from build123d import *

# Parameters (mm, degrees)
SKETCH_W     = 42
SKETCH_H     = 42
PAD_DEPTH    = 47
SKETCH001_R  = 1.5
POCKET_DEPTH = 4.5
SKETCH002_R  = 11
PAD001_DEPTH = 2
SKETCH003_R  = 2.5
PAD002_DEPTH = 22


with BuildPart() as part:
    # Sketch → Pad (new body)
    with BuildSketch(Plane.XY):
        Rectangle(SKETCH_W, SKETCH_H)
    extrude(amount=PAD_DEPTH)

    # Sketch001 (on Face6 of Pad) → Pocket (cut)
    with BuildSketch(Plane.XY.offset(47)):
        with Locations((-15.5, 15.5)):
            Circle(SKETCH001_R)
        with Locations((15.5, 16)):
            Circle(SKETCH001_R)
        with Locations((15.5, -15)):
            Circle(SKETCH001_R)
        with Locations((-15.5, -15.5)):
            Circle(SKETCH001_R)
    extrude(amount=-POCKET_DEPTH, mode=Mode.SUBTRACT)

    # Sketch002 (on Face5 of Pocket) → Pad001 (join)
    with BuildSketch(Plane.XY.offset(47)):
        Circle(SKETCH002_R)
    extrude(amount=PAD001_DEPTH)

    # Sketch003 (on Face13 of Pad001) → Pad002 (join)
    with BuildSketch(Plane.XY.offset(49)):
        Circle(SKETCH003_R)
    extrude(amount=PAD002_DEPTH)


solid = part.part
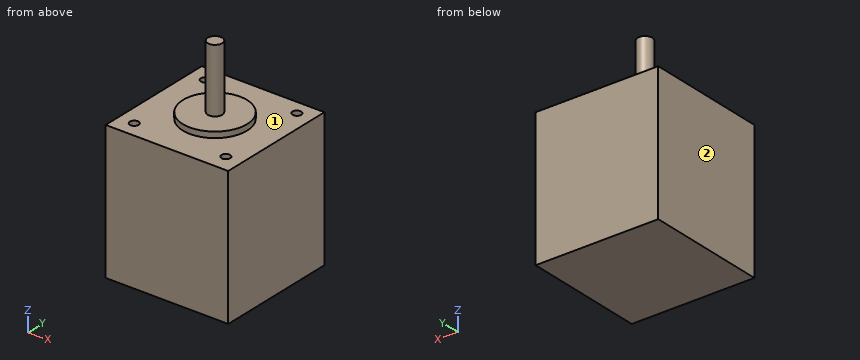
The listing builds one solid part. Answer for the finished solid, in the listing's coordinates (mm). Face numbers are marked on the shaded views. A direction names the side the tool comes from. Round coordinates to 2 decimals unless told otherwise and drop trailing zeros. Order: outer loops, then holes, each group sorted by start corner. A loop starts at its lowest first (then second) coordinate and runs counter-clockwise, first axis right, second up. Notation, with made-up numbers: (8.5, 37.5) -> (29.5, 37.5) arc R16 cw to (29.5, 62.5) -> close; hole circle Ø9 at (25, 17.5). An arc over 180 degrees is marked (long way). Write each question's results on one line, items separated by ' | '. Start each with the question number.
Q1. Find section A-A (y = 0). Determine the outline of the cut face in (x, z), then the cut area to 3 significant figures.
Q2. Which of the six approach directions +Z, -Z, +X, -X, +Y, -Y give full straight-line access (tool end or side, diameter ignored) to the marked faces 1 and 2?
Q3. Each of these flat-tipped pins is pushed along its axis until it touches: pin 1 (1.8 mm diameter, centred on x = -15.5, y = -15.5, fed in from +Z); pin 2 (3.5 mm diameter, centred on x = 16, y = -14.5, fed in from +Z). Where does it stop, or does it pass through?
Q4. Straight lines are drawn through the part: probe 1 along Y at (x, z) = (-15.5, 45.15); probe 2 along X at (y, z) = (15, 45); probe 3 along Z at (x, y) = (9, -15). For each, find the intervals that lie inside material, in ascending order. Write a range as from..to.
Q5. Find section C-C (z = 58). Determine the outline of the cut face in (x, y), then the cut area to 3 significant figures.
Q6. Find section D-D (x = 5). Determine the outline of the cut face in (y, z), then the cut area to 3 significant figures.
Worked answers:
1) outline: (-21, 0) -> (21, 0) -> (21, 47) -> (11, 47) -> (11, 49) -> (2.5, 49) -> (2.5, 71) -> (-2.5, 71) -> (-2.5, 49) -> (-11, 49) -> (-11, 47) -> (-21, 47) -> close | area: 2,130 mm2
2) face 1: +Z | face 2: +Z, -Z, -X, +Y, -Y
3) pin 1: stops at z = 42.5 | pin 2: stops at z = 47
4) probe 1: y = -21..-17, -14..14, 17..21 | probe 2: x = -21..-16.91, -14.09..14.38, 16.62..21 | probe 3: z = 0..47
5) outline: circle Ø5 at (0, 0) | area: 19.6 mm2
6) outline: (-21, 0) -> (21, 0) -> (21, 47) -> (9.8, 47) -> (9.8, 49) -> (-9.8, 49) -> (-9.8, 47) -> (-21, 47) -> close | area: 2,010 mm2
